Part model, mm, in its own coordinate system. Round coordinates to 2 decimals unless told otherwise and drop trailing zeros. Loops run counter-clockwise (first coordinate to the right, second up) from the corner with the lowest first, then second, coordinate; pieces in that order, holes last.
1) Drop a flat-ended pin along its axis: P1, Ø3.5, axis at x = -141, y = 0.5, coming from the +Z side. Give the stop position or say it passes through.
2) Band-saw the part on B-B, the plane y = -130. Write the cut outline in (x, z).
3) Band-saw the part on C-C, the plane z = 3.25. State how many separate pieces and enclosed holes the cut face has, then the cut area to 3 significant figures.
4) Probe line 1 (X direction, y = 15, z = 5.75); line 2 (X direction, y = 155.5, z = 2.1); line 3 (Y direction, x = 175, z = 3.75). List the from-to ranges inside material, lowest first.
5) Band-saw the part on A-A, the plane x = 110. Write the cut outline in (y, z).
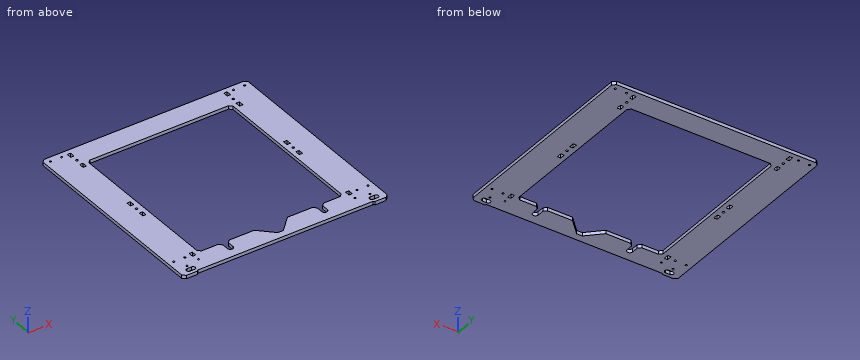
from build123d import *

# Parameters (mm, degrees)
SZKIC1_W                    = 370
SZKIC1_H                    = 370
SZKIC1_W_2                  = 260
SZKIC1_H_2                  = 290
DODANIE_WYCI_GNI_CIE1_DEPTH = 6
WYTNIJ_WYCI_GNI_CIE1_REACH  = 263.698
SFAZOWANIE1_SIZE            = 5
WYTNIJ_WYCI_GNI_CIE2_REACH  = 263.698
WYTNIJ_WYCI_GNI_CIE3_REACH  = 263.698
SZKIC4_R                    = 2
SZKIC4_R_2                  = 1.5
SZKIC4_W                    = 6
SZKIC4_H                    = 9
WYTNIJ_WYCI_GNI_CIE4_REACH  = 263.698
SZKIC5_R                    = 1.7
WYTNIJ_WYCI_GNI_CIE5_REACH  = 263.698


with BuildPart() as part:
    # Szkic1 → Dodanie-wyci_gni_cie1 (new body)
    with BuildSketch(Plane.XY):
        Rectangle(SZKIC1_W, SZKIC1_H)
        Rectangle(SZKIC1_W_2, SZKIC1_H_2, mode=Mode.SUBTRACT)
    extrude(amount=DODANIE_WYCI_GNI_CIE1_DEPTH)

    # Szkic2 → Wytnij-wyci_gni_cie1 (cut, up to next)
    with BuildSketch(Plane.XY.offset(6), mode=Mode.PRIVATE) as wytnij_wyci_gni_cie1_sk1:
        with BuildLine():
            Line((90, -145), (90, -162))
            ThreePointArc((90, -162), (85, -167), (80, -162))
            Line((80, -162), (80, -145))
            Line((80, -145), (90, -145))
        make_face()
    wytnij_wyci_gni_cie1_tool1 = extrude(wytnij_wyci_gni_cie1_sk1.sketch, amount=-WYTNIJ_WYCI_GNI_CIE1_REACH, mode=Mode.PRIVATE) & part.part
    # Szkic2 → Wytnij-wyci_gni_cie1 (cut, up to next)
    with BuildSketch(Plane.XY.offset(6), mode=Mode.PRIVATE) as wytnij_wyci_gni_cie1_sk2:
        Polygon((-5, -170), (5, -170), (30, -145), (-30, -145), align=None)
    wytnij_wyci_gni_cie1_tool2 = extrude(wytnij_wyci_gni_cie1_sk2.sketch, amount=-WYTNIJ_WYCI_GNI_CIE1_REACH, mode=Mode.PRIVATE) & part.part
    # Szkic2 → Wytnij-wyci_gni_cie1 (cut, up to next)
    with BuildSketch(Plane.XY.offset(6), mode=Mode.PRIVATE) as wytnij_wyci_gni_cie1_sk3:
        with BuildLine():
            Line((-90, -145), (-90, -162))
            ThreePointArc((-90, -162), (-85, -167), (-80, -162))
            Line((-80, -162), (-80, -145))
            Line((-80, -145), (-90, -145))
        make_face()
    wytnij_wyci_gni_cie1_tool3 = extrude(wytnij_wyci_gni_cie1_sk3.sketch, amount=-WYTNIJ_WYCI_GNI_CIE1_REACH, mode=Mode.PRIVATE) & part.part
    add(wytnij_wyci_gni_cie1_tool1.solids().sort_by_distance((85, -155.493251, 6))[0], mode=Mode.SUBTRACT)
    add(wytnij_wyci_gni_cie1_tool2.solids().sort_by_distance((0, -154.52381, 6))[0], mode=Mode.SUBTRACT)
    add(wytnij_wyci_gni_cie1_tool3.solids().sort_by_distance((-85, -155.493251, 6))[0], mode=Mode.SUBTRACT)

    # Sfazowanie1
    sfazowanie1_edges = [part.edges().sort_by_distance(p)[0] for p in [
        (-130, 145, 3),
        (-130, -145, 3),
        (130, -145, 3),
        (130, 145, 3),
        (80, -145, 3),
        (90, -145, 3),
        (-90, -145, 3),
        (-80, -145, 3),
        (185, -185, 3),
        (-185, -185, 3),
        (-185, 185, 3),
        (185, 185, 3),
    ]]
    chamfer(sfazowanie1_edges, length=SFAZOWANIE1_SIZE)

    # Szkic3 → Wytnij-wyci_gni_cie2 (cut, up to next)
    with BuildSketch(Plane.XY.offset(6), mode=Mode.PRIVATE) as wytnij_wyci_gni_cie2_sk1:
        Polygon((-158, -183), (158, -183), (160, -185), (-160, -185), align=None)
    wytnij_wyci_gni_cie2_tool1 = extrude(wytnij_wyci_gni_cie2_sk1.sketch, amount=-WYTNIJ_WYCI_GNI_CIE2_REACH, mode=Mode.PRIVATE) & part.part
    add(wytnij_wyci_gni_cie2_tool1.solids().sort_by_distance((0, -184.002096, 6))[0], mode=Mode.SUBTRACT)

    # Szkic4 → Wytnij-wyci_gni_cie3 (cut, up to next)
    with BuildSketch(Plane.XY.offset(6), mode=Mode.PRIVATE) as wytnij_wyci_gni_cie3_sk1:
        with Locations((141, 155.5)):
            Circle(SZKIC4_R)
    wytnij_wyci_gni_cie3_tool1 = extrude(wytnij_wyci_gni_cie3_sk1.sketch, amount=-WYTNIJ_WYCI_GNI_CIE3_REACH, mode=Mode.PRIVATE) & part.part
    # Szkic4 → Wytnij-wyci_gni_cie3 (cut, up to next)
    with BuildSketch(Plane.XY.offset(6), mode=Mode.PRIVATE) as wytnij_wyci_gni_cie3_sk2:
        with Locations((141, 0.5)):
            Circle(SZKIC4_R)
    wytnij_wyci_gni_cie3_tool2 = extrude(wytnij_wyci_gni_cie3_sk2.sketch, amount=-WYTNIJ_WYCI_GNI_CIE3_REACH, mode=Mode.PRIVATE) & part.part
    # Szkic4 → Wytnij-wyci_gni_cie3 (cut, up to next)
    with BuildSketch(Plane.XY.offset(6), mode=Mode.PRIVATE) as wytnij_wyci_gni_cie3_sk3:
        with Locations((141, -160.5)):
            Circle(SZKIC4_R_2)
    wytnij_wyci_gni_cie3_tool3 = extrude(wytnij_wyci_gni_cie3_sk3.sketch, amount=-WYTNIJ_WYCI_GNI_CIE3_REACH, mode=Mode.PRIVATE) & part.part
    # Szkic4 → Wytnij-wyci_gni_cie3 (cut, up to next)
    with BuildSketch(Plane.XY.offset(6), mode=Mode.PRIVATE) as wytnij_wyci_gni_cie3_sk4:
        with Locations((141, 171.5)):
            Rectangle(SZKIC4_W, SZKIC4_H)
    wytnij_wyci_gni_cie3_tool4 = extrude(wytnij_wyci_gni_cie3_sk4.sketch, amount=-WYTNIJ_WYCI_GNI_CIE3_REACH, mode=Mode.PRIVATE) & part.part
    # Szkic4 → Wytnij-wyci_gni_cie3 (cut, up to next)
    with BuildSketch(Plane.XY.offset(6), mode=Mode.PRIVATE) as wytnij_wyci_gni_cie3_sk5:
        with Locations((141, 139.5)):
            Rectangle(SZKIC4_W, SZKIC4_H)
    wytnij_wyci_gni_cie3_tool5 = extrude(wytnij_wyci_gni_cie3_sk5.sketch, amount=-WYTNIJ_WYCI_GNI_CIE3_REACH, mode=Mode.PRIVATE) & part.part
    # Szkic4 → Wytnij-wyci_gni_cie3 (cut, up to next)
    with BuildSketch(Plane.XY.offset(6), mode=Mode.PRIVATE) as wytnij_wyci_gni_cie3_sk6:
        with Locations((141, -15.5)):
            Rectangle(SZKIC4_W, SZKIC4_H)
    wytnij_wyci_gni_cie3_tool6 = extrude(wytnij_wyci_gni_cie3_sk6.sketch, amount=-WYTNIJ_WYCI_GNI_CIE3_REACH, mode=Mode.PRIVATE) & part.part
    # Szkic4 → Wytnij-wyci_gni_cie3 (cut, up to next)
    with BuildSketch(Plane.XY.offset(6), mode=Mode.PRIVATE) as wytnij_wyci_gni_cie3_sk7:
        with Locations((141, 16.5)):
            Rectangle(SZKIC4_W, SZKIC4_H)
    wytnij_wyci_gni_cie3_tool7 = extrude(wytnij_wyci_gni_cie3_sk7.sketch, amount=-WYTNIJ_WYCI_GNI_CIE3_REACH, mode=Mode.PRIVATE) & part.part
    # Szkic4 → Wytnij-wyci_gni_cie3 (cut, up to next)
    with BuildSketch(Plane.XY.offset(6), mode=Mode.PRIVATE) as wytnij_wyci_gni_cie3_sk8:
        with Locations((141, -144.5)):
            Rectangle(SZKIC4_W, SZKIC4_H)
    wytnij_wyci_gni_cie3_tool8 = extrude(wytnij_wyci_gni_cie3_sk8.sketch, amount=-WYTNIJ_WYCI_GNI_CIE3_REACH, mode=Mode.PRIVATE) & part.part
    wytnij_wyci_gni_cie3_1 = wytnij_wyci_gni_cie3_tool1.solids().sort_by_distance((141, 155.5, 6))[0]
    add(wytnij_wyci_gni_cie3_1, mode=Mode.SUBTRACT)
    wytnij_wyci_gni_cie3_2 = wytnij_wyci_gni_cie3_tool2.solids().sort_by_distance((141, 0.5, 6))[0]
    add(wytnij_wyci_gni_cie3_2, mode=Mode.SUBTRACT)
    wytnij_wyci_gni_cie3_3 = wytnij_wyci_gni_cie3_tool3.solids().sort_by_distance((141, -160.5, 6))[0]
    add(wytnij_wyci_gni_cie3_3, mode=Mode.SUBTRACT)
    wytnij_wyci_gni_cie3_4 = wytnij_wyci_gni_cie3_tool4.solids().sort_by_distance((141, 171.5, 6))[0]
    add(wytnij_wyci_gni_cie3_4, mode=Mode.SUBTRACT)
    wytnij_wyci_gni_cie3_5 = wytnij_wyci_gni_cie3_tool5.solids().sort_by_distance((141, 139.5, 6))[0]
    add(wytnij_wyci_gni_cie3_5, mode=Mode.SUBTRACT)
    wytnij_wyci_gni_cie3_6 = wytnij_wyci_gni_cie3_tool6.solids().sort_by_distance((141, -15.5, 6))[0]
    add(wytnij_wyci_gni_cie3_6, mode=Mode.SUBTRACT)
    wytnij_wyci_gni_cie3_7 = wytnij_wyci_gni_cie3_tool7.solids().sort_by_distance((141, 16.5, 6))[0]
    add(wytnij_wyci_gni_cie3_7, mode=Mode.SUBTRACT)
    wytnij_wyci_gni_cie3_8 = wytnij_wyci_gni_cie3_tool8.solids().sort_by_distance((141, -144.5, 6))[0]
    add(wytnij_wyci_gni_cie3_8, mode=Mode.SUBTRACT)
    wytnij_wyci_gni_cie3 = wytnij_wyci_gni_cie3_1 + wytnij_wyci_gni_cie3_2 + wytnij_wyci_gni_cie3_3 + wytnij_wyci_gni_cie3_4 + wytnij_wyci_gni_cie3_5 + wytnij_wyci_gni_cie3_6 + wytnij_wyci_gni_cie3_7 + wytnij_wyci_gni_cie3_8  # Wytnij-wyci_gni_cie3 as one shape, for the pattern or mirror that repeats it

    # Szkic5 → Wytnij-wyci_gni_cie4 (cut, up to next)
    with BuildSketch(Plane.XY.offset(6), mode=Mode.PRIVATE) as wytnij_wyci_gni_cie4_sk1:
        with Locations((175, 175)):
            Circle(SZKIC5_R)
    wytnij_wyci_gni_cie4_tool1 = extrude(wytnij_wyci_gni_cie4_sk1.sketch, amount=-WYTNIJ_WYCI_GNI_CIE4_REACH, mode=Mode.PRIVATE) & part.part
    # Szkic5 → Wytnij-wyci_gni_cie4 (cut, up to next)
    with BuildSketch(Plane.XY.offset(6), mode=Mode.PRIVATE) as wytnij_wyci_gni_cie4_sk2:
        with Locations((155, 175)):
            Circle(SZKIC5_R)
    wytnij_wyci_gni_cie4_tool2 = extrude(wytnij_wyci_gni_cie4_sk2.sketch, amount=-WYTNIJ_WYCI_GNI_CIE4_REACH, mode=Mode.PRIVATE) & part.part
    # Szkic5 → Wytnij-wyci_gni_cie4 (cut, up to next)
    with BuildSketch(Plane.XY.offset(6), mode=Mode.PRIVATE) as wytnij_wyci_gni_cie4_sk3:
        with Locations((175, -145)):
            Circle(SZKIC5_R)
    wytnij_wyci_gni_cie4_tool3 = extrude(wytnij_wyci_gni_cie4_sk3.sketch, amount=-WYTNIJ_WYCI_GNI_CIE4_REACH, mode=Mode.PRIVATE) & part.part
    # Szkic5 → Wytnij-wyci_gni_cie4 (cut, up to next)
    with BuildSketch(Plane.XY.offset(6), mode=Mode.PRIVATE) as wytnij_wyci_gni_cie4_sk4:
        with Locations((155, -145)):
            Circle(SZKIC5_R)
    wytnij_wyci_gni_cie4_tool4 = extrude(wytnij_wyci_gni_cie4_sk4.sketch, amount=-WYTNIJ_WYCI_GNI_CIE4_REACH, mode=Mode.PRIVATE) & part.part
    # Szkic5 → Wytnij-wyci_gni_cie4 (cut, up to next)
    with BuildSketch(Plane.XY.offset(6), mode=Mode.PRIVATE) as wytnij_wyci_gni_cie4_sk5:
        with Locations((165, -165)):
            Circle(SZKIC5_R)
    wytnij_wyci_gni_cie4_tool5 = extrude(wytnij_wyci_gni_cie4_sk5.sketch, amount=-WYTNIJ_WYCI_GNI_CIE4_REACH, mode=Mode.PRIVATE) & part.part
    wytnij_wyci_gni_cie4_1 = wytnij_wyci_gni_cie4_tool1.solids().sort_by_distance((175, 175, 6))[0]
    add(wytnij_wyci_gni_cie4_1, mode=Mode.SUBTRACT)
    wytnij_wyci_gni_cie4_2 = wytnij_wyci_gni_cie4_tool2.solids().sort_by_distance((155, 175, 6))[0]
    add(wytnij_wyci_gni_cie4_2, mode=Mode.SUBTRACT)
    wytnij_wyci_gni_cie4_3 = wytnij_wyci_gni_cie4_tool3.solids().sort_by_distance((175, -145, 6))[0]
    add(wytnij_wyci_gni_cie4_3, mode=Mode.SUBTRACT)
    wytnij_wyci_gni_cie4_4 = wytnij_wyci_gni_cie4_tool4.solids().sort_by_distance((155, -145, 6))[0]
    add(wytnij_wyci_gni_cie4_4, mode=Mode.SUBTRACT)
    wytnij_wyci_gni_cie4_5 = wytnij_wyci_gni_cie4_tool5.solids().sort_by_distance((165, -165, 6))[0]
    add(wytnij_wyci_gni_cie4_5, mode=Mode.SUBTRACT)
    wytnij_wyci_gni_cie4 = wytnij_wyci_gni_cie4_1 + wytnij_wyci_gni_cie4_2 + wytnij_wyci_gni_cie4_3 + wytnij_wyci_gni_cie4_4 + wytnij_wyci_gni_cie4_5  # Wytnij-wyci_gni_cie4 as one shape, for the pattern or mirror that repeats it

    # Szkic6 → Wytnij-wyci_gni_cie5 (cut, up to next)
    with BuildSketch(Plane(origin=(0, 0, 0), x_dir=(-1, 0, 0), z_dir=(0, 0, -1)), mode=Mode.PRIVATE) as wytnij_wyci_gni_cie5_sk1:
        with BuildLine():
            Line((161, -171), (169, -171))
            ThreePointArc((169, -171), (173, -175), (169, -179))
            Line((169, -179), (161, -179))
            ThreePointArc((161, -179), (157, -175), (161, -171))
        make_face()
    wytnij_wyci_gni_cie5_tool1 = extrude(wytnij_wyci_gni_cie5_sk1.sketch, amount=-WYTNIJ_WYCI_GNI_CIE5_REACH, mode=Mode.PRIVATE) & part.part
    wytnij_wyci_gni_cie5 = wytnij_wyci_gni_cie5_tool1.solids().sort_by_distance((-165, -175, 0))[0]
    add(wytnij_wyci_gni_cie5, mode=Mode.SUBTRACT)

    # Lustro1: Wytnij-wyci_gni_cie3, Wytnij-wyci_gni_cie4, Wytnij-wyci_gni_cie5 across plane
    add(wytnij_wyci_gni_cie3.mirror(Plane(origin=(0, 0, 0), x_dir=(0, 0, 1), z_dir=(1, 0, 0))), mode=Mode.SUBTRACT)
    add(wytnij_wyci_gni_cie4.mirror(Plane(origin=(0, 0, 0), x_dir=(0, 0, 1), z_dir=(1, 0, 0))), mode=Mode.SUBTRACT)
    add(wytnij_wyci_gni_cie5.mirror(Plane(origin=(0, 0, 0), x_dir=(0, 0, 1), z_dir=(1, 0, 0))), mode=Mode.SUBTRACT)


solid = part.part
Reported:
1. P1: passes through
2. outline: (-185, 0) - (-130, 0) - (-130, 6) - (-185, 6) - close; (130, 0) - (185, 0) - (185, 6) - (130, 6) - close
3. separate pieces: 1
3. enclosed holes: 29
3. area: 58,600 mm2
4. line 1: x = -185 to -144, -138 to -130, 130 to 138, 144 to 185
4. line 2: x = -185 to -143, -139 to 139, 143 to 185
4. line 3: y = -185 to -146.7, -143.3 to 173.3, 176.7 to 185
5. outline: (-183, 0) - (-145, 0) - (-145, 6) - (-183, 6) - close; (145, 0) - (185, 0) - (185, 6) - (145, 6) - close
